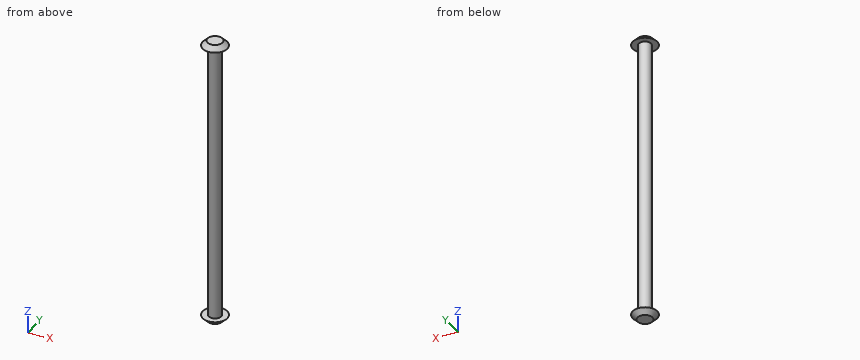
from build123d import *

# Parameters (mm, degrees)
SKETCH1_R                = 3.175
BOSS_EXTRUDE1_DEPTH      = 144.78
SKETCH2_R                = 6.35
BOSS_EXTRUDE2_DEPTH      = 2.54
CHAMFER1_SIZE            = 2.54
CHAMFER1_OF_MIRROR1_SIZE = 2.54


with BuildPart() as part:
    # Sketch1 → Boss-Extrude1 (new body)
    with BuildSketch(Plane.XY):
        Circle(SKETCH1_R)
    extrude(amount=BOSS_EXTRUDE1_DEPTH)

    # Sketch2 → Boss-Extrude2 (add)
    with BuildSketch(Plane.XY.offset(144.78)):
        Circle(SKETCH2_R)
    boss_extrude2 = extrude(amount=BOSS_EXTRUDE2_DEPTH)

    # Chamfer1
    chamfer1_edges = [part.edges().sort_by_distance(p)[0] for p in [
        (-6.35, 0, 147.32),
    ]]
    chamfer(chamfer1_edges, length=CHAMFER1_SIZE - 0.0001)  # a hair under: the kernel refuses the full size

    # Mirror1: Boss-Extrude2 across plane
    add(boss_extrude2.mirror(Plane(origin=(0, 0, 72.39), x_dir=(1, 0, 0), z_dir=(0, 0, -1))))

    # Chamfer1 of Mirror1
    chamfer1_of_mirror1_edges = [part.edges().sort_by_distance(p)[0] for p in [
        (-6.35, 0, -2.54),
    ]]
    chamfer(chamfer1_of_mirror1_edges, length=CHAMFER1_OF_MIRROR1_SIZE - 0.0001)  # a hair under: the kernel refuses the full size


solid = part.part
CAD build for the part. Positions are in the model's coordinates, mm. Give positions to 0.01 mm unless a question says otherwise; leave off trailing zeros. Loops run counter-clockwise (first coordinate to the right, second up) from the corner with the lowest first, then second, coordinate; pieces in that order, holes last. Notation, with made-up numbers: M 53.25,-39 L 102.25,-39 A26 cw 102.25,-10 Z; hole C 71.25,21 d6. An arc over 180 degrees is marked long. One line per question, with ' | ' between items. Start each with the question number.
1. Probe L1, parallel to Y at x = -0.25, z = 104; L2, parallel to Z at x = -5, y = 0.25; L3, parallel to Z at x = -0.5, y = 4.25. List the from-to ranges inside material, lowest first. Write a range as from..to.
2. Saw through at C-C on z = 121.5. Give the cut face in (x, y) (3 decimals), plus the area to 3 significant figures.
3. Flat gauge pins, fed straight in: pin 1 (2 mm diameter, centred on x = 3, y = -4.5, fed in from +Z); pin 2 (1.5 mm diameter, centred on x = 2.5, z = 30, fed in from +Y); pin 3 (4 mm diameter, centred on x = -0.5, z = 115, fed in from +Y) (3 decimals). Where does each tip first touch, or does it go through?
Result sheet:
1) L1: y = -3.17..3.17 | L2: z = -1.34..0, 144.78..146.12 | L3: z = -2.07..0, 144.78..146.85
2) outline: C 0,0 d6.35 | area: 31.7 mm^2
3) pin 1: stops at z = 146.72 | pin 2: stops at y = 2.65 | pin 3: stops at y = 3.175
